Could you check a few things on this model? Use its own coordinates, in mm. Face numbers are marked on the shaded views. A direction names the side the tool comes from. Round coordinates to 2 decimals unless told otherwise and drop trailing zeros. Loops run counter-clockwise (first coordinate to the right, second up) from the corner with the lowest first, then second, coordinate; pieces in that order, holes last.
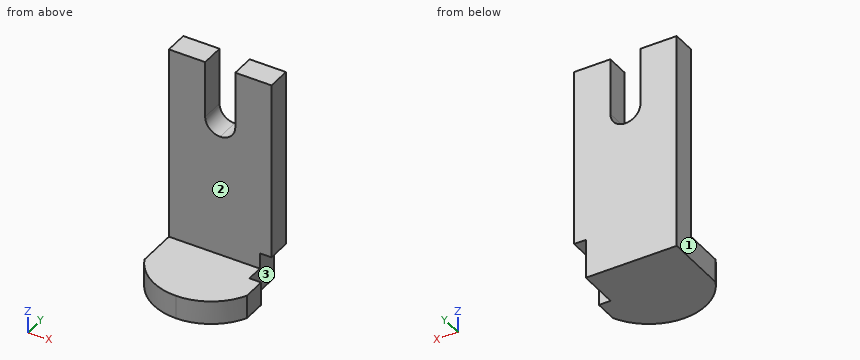
from build123d import *

# Parameters (mm, degrees)
F1_DEPTH      = 118.364
F2_W          = 68.2598565102
F2_H          = 105.664
F3_DEPTH      = 27.844343094
F3_DEPTH_BACK = 27.844343094
F4_W          = 9.2177082181
F4_H          = 8.6436167687
F5_DEPTH      = 6.35
F7_DEPTH      = 51.7396268929


with BuildPart() as f1:
    # F0 (on Top) → F1 (new body)
    with BuildSketch(Plane.XY):
        with BuildLine():
            Line((27.843343094, 0), (0, 0))
            Line((0, 0), (-27.843343094, 0))
            Line((-27.843343094, 0), (-27.843343094, -34.4115048647))
            ThreePointArc((-27.843343094, -34.4115048647), (-16.3972628236, -47.053149323), (0, -51.7386268929))
            ThreePointArc((0, -51.7386268929), (16.3972628236, -47.053149323), (27.843343094, -34.4115048647))
            Line((27.843343094, -34.4115048647), (27.843343094, 0))
        make_face()
    extrude(amount=F1_DEPTH)

    # F2 (on Right) → F3 (cut, two sides)
    with BuildSketch(Plane.YZ) as f3_sk:
        with Locations((-46.8299282551, 65.532)):
            Rectangle(F2_W, F2_H)
    extrude(amount=-F3_DEPTH, mode=Mode.SUBTRACT)
    extrude(f3_sk.sketch, amount=F3_DEPTH_BACK, mode=Mode.SUBTRACT)

    # F4 (on face) → F5 (cut)
    with BuildSketch(Plane.YZ.offset(27.843343094)):
        with Locations((-17.308854109, 17.0218083844)):
            Rectangle(F4_W, F4_H)
        Polygon((-21.9177082181, 0), (0, 0), (0, 21.3436167687), (-12.7, 21.3436167687), (-12.7, 12.7), (-21.9177082181, 12.7), align=None)
    extrude(amount=-F5_DEPTH, mode=Mode.SUBTRACT)

    # F6 (on face) → F7 (cut, through all)
    with BuildSketch(Plane(origin=(0, 0, 0), x_dir=(-1, 0, 0), z_dir=(0, 1, 0))):
        with BuildLine():
            Line((8.167100139, 118.364), (0, 118.364))
            Line((0, 118.364), (-8.167100139, 118.364))
            Line((-8.167100139, 118.364), (-8.167100139, 87.4478146434))
            ThreePointArc((-8.167100139, 87.4478146434), (-5.7750118909, 81.6728027525), (0, 79.2807145044))
            ThreePointArc((0, 79.2807145044), (5.7750118909, 81.6728027525), (8.167100139, 87.4478146434))
            Line((8.167100139, 87.4478146434), (8.167100139, 118.364))
        make_face()
    extrude(amount=-F7_DEPTH, mode=Mode.SUBTRACT)


solid = f1.part
Item 1: For the marked faces 1, 2 and 3, which set-ups out of +Z, -Z, +X, -X, +Y, -Y let a thin tool reach every point of the face, with its end or its side?
Results list:
face 1: +Z, -Z, -X, +Y, -Y
face 2: +Z, +X, -X, -Y
face 3: -Z, +X, +Y
Item 2: If we section it at A-A, the plane y = -2.5: Please give me the cut outline in (x, z).
Results list:
outline: (-27.84, 0) - (21.49, 0) - (21.49, 21.34) - (27.84, 21.34) - (27.84, 118.36) - (8.17, 118.36) - (8.17, 87.45) arc R8.17 cw to (-8.17, 87.45) - (-8.17, 118.36) - (-27.84, 118.36) - close
Item 3: If we section it at B-B, the plane z = 9: Please give me the cut outline in (x, y), then the cut area to 3 significant figures.
Results list:
outline: (-27.84, -34.41) arc R31.03 ccw to (27.84, -34.41) - (27.84, -21.92) - (21.49, -21.92) - (21.49, 0) - (-27.84, 0) - close
area: 2,470 mm2
Item 4: If we section it at D-D, the plane z = 26: Please give me the cut outline in (x, y).
Results list:
outline: (-27.84, -12.7) - (27.84, -12.7) - (27.84, 0) - (-27.84, 0) - close
Item 5: If we section it at C-C, the plane x = -9.5: Please give me the cut outline in (y, z).
Results list:
outline: (-50.25, 0) - (0, 0) - (0, 118.36) - (-12.7, 118.36) - (-12.7, 12.7) - (-50.25, 12.7) - close
Item 6: If I drill on line 1 along Y through (x, z) = (-25, 102); line 2 along Z through (x, y) = (-22, -33); line 3 along X through (y, z) = (-3, 10), over which ranges is the centre line in solid material (lowest first)?
Results list:
line 1: y = -12.7 to 0
line 2: z = 0 to 12.7
line 3: x = -27.84 to 21.49
Item 7: Will these pins go through, and if not, where does the flat tip stop? pin 1 (3 mm diameter, centred on x = 1.5, y = -35.5, fed in from +Z); pin 2 (6 mm diameter, centred on x = -3.5, z = 58.5, fed in from -Y); pin 3 (2 mm diameter, centred on x = 18, y = -32, fed in from -Z); pin 4 (8 mm diameter, centred on y = -40, z = 19.5, fed in from -X).
Results list:
pin 1: stops at z = 12.7
pin 2: stops at y = -12.7
pin 3: stops at z = 0
pin 4: passes through
